```python
from build123d import *

# Parameters (mm, degrees)
PAD021_DEPTH = 7.4
PAD022_DEPTH = 10.8
SKETCH051_R  = 6.1
PAD023_DEPTH = 3.5
SKETCH052_R  = 5
PAD024_DEPTH = 4


with BuildPart() as part:
    # Sketch049 → Pad021 (new body)
    with BuildSketch(Plane.XY):
        with BuildLine():
            ThreePointArc((2.2326625821, -7.7862197371), (8.1, 0), (2.2326625821, 7.7862197371))
            Line((1.7916428128, 6.2482010236), (2.2326625821, 7.7862197371))
            ThreePointArc((1.7916428128, -6.2482010236), (6.5, 0), (1.7916428128, 6.2482010236))
            Line((1.7916428128, -6.2482010236), (2.2326625821, -7.7862197371))
        make_face()
    extrude(amount=PAD021_DEPTH)

    # Sketch050 (on Face6 of Pad021) → Pad022 (join)
    with BuildSketch(Plane.XY.offset(7.4)):
        with BuildLine():
            ThreePointArc((10.5423930727, 6.7162451043), (-12.5, 0), (10.5423930727, -6.7162451043))
            Line((10.5423930727, -6.7162451043), (7.253166434, -4.6207766318))
            ThreePointArc((7.253166434, -4.6207766318), (8.6, 0), (7.253166434, 4.6207766318))
            Line((10.5423930727, 6.7162451043), (7.253166434, 4.6207766318))
        make_face()
        with BuildLine():
            ThreePointArc((2.4256087312, 8.4591029243), (-8.8, 0), (2.4256087312, -8.4591029243))
            Line((1.7916428128, -6.2482010236), (2.4256087312, -8.4591029243))
            ThreePointArc((1.7916428128, -6.2482010236), (6.5, 0), (1.7916428128, 6.2482010236))
            Line((1.7916428128, 6.2482010236), (2.4256087312, 8.4591029243))
        make_face(mode=Mode.SUBTRACT)
    extrude(amount=PAD022_DEPTH)

    # Sketch051 (on Face10 of Pad022) → Pad023 (join)
    with BuildSketch(Plane.XY.offset(18.2)):
        with BuildLine():
            ThreePointArc((10.5423930727, 6.7162451043), (-12.5, 0), (10.5423930727, -6.7162451043))
            Line((10.5423930727, -6.7162451043), (7.253166434, -4.6207766318))
            ThreePointArc((7.253166434, -4.6207766318), (8.6, 0), (7.253166434, 4.6207766318))
            Line((10.5423930727, 6.7162451043), (7.253166434, 4.6207766318))
        make_face()
        Circle(SKETCH051_R, mode=Mode.SUBTRACT)
    extrude(amount=PAD023_DEPTH)

    # Sketch052 (on Face21 of Pad023) → Pad024 (join)
    with BuildSketch(Plane.XY.offset(21.7)):
        with BuildLine():
            ThreePointArc((10.5423930727, 6.7162451043), (-12.5, 0), (10.5423930727, -6.7162451043))
            Line((10.5423930727, -6.7162451043), (7.253166434, -4.6207766318))
            ThreePointArc((7.253166434, -4.6207766318), (8.6, 0), (7.253166434, 4.6207766318))
            Line((10.5423930727, 6.7162451043), (7.253166434, 4.6207766318))
        make_face()
        Circle(SKETCH052_R, mode=Mode.SUBTRACT)
    extrude(amount=PAD024_DEPTH)


with BuildPart() as part_1:
    # Body006 placement: moved
    add(part.part.moved(Location((0, 0, 2.2))))


solid = part_1.part
```
Check sheet for the modelled part. Datum: model origin and axes. Units: mm. A direction names the side the tool comes from. Coordinates: 2 decimals unless noted, no trailing zeros. Loops run counter-clockwise (first coordinate to the right, second up) from the corner with the lowest first, then second, coordinate; pieces in that order, holes last.
1) Sectioned sample at B-B (x = 0). Record the boundary of the cut face in (y, z).
2) Access from +Z, -Z, +X, -X, +Y, -Y to the whole of each face (thin tool, end or side, straight path). Record for faces 1 (the face through (8.1, -0.1, 5.8)), 2 (the face through (8.921, -5.683, 18.622)), 3 (the face through (6.5, -0.1, 11.2)).
3) Release check for a two-part mould opening along Y. For faces 4 (the face through (7, 0, 2.2)), 5 (the face through (8.6, -0.1, 18.6)), 6 (the face through (-12.49, 0.45, 18.62)), 7 (the face through (-6.3, -1.3, 20.4)) record: released by +Y, released by -Y, zero draft, split by the parting line, or undercut.
4) Sectioned sample at C-C (z = 12.25). Record the boundary of the cut face in (x, y).
5) Gauge pin test, flat ends, axial feed: pin 1 (8 mm diameter, centred on x = -0.5, y = 2.5, fed in from -Z); pin 2 (1.5 mm diameter, centred on x = -4, z = 20.5, fed in from -Y); pin 3 (1.5 mm diameter, centred on y = -1.5, z = 6, fed in from +X); pin 4 (6 mm diameter, centred on x = 0, y = -0.5, fed in from -Z). Record the tip position at first contact, or that the pin passes through.
6) Sectioned sample at A-A (y = 0). Record the boundary of the cut face in (x, z).
7) Sectioned sample at D-D (z = 21.25). Record the boundary of the cut face in (x, y), and give its area (3 significant figures).
8) Material ranges on probe 1 along Y at (x, z) = (0, 15); probe 2 along Y at (x, z) = (0, 26); probe 3 along X at (y, z) = (2.25, 16), recorded low to high.
Check sheet entries:
1. outline: (-12.5, 9.6) - (-8.8, 9.6) - (-8.8, 20.4) - (-6.1, 20.4) - (-6.1, 23.9) - (-5, 23.9) - (-5, 27.9) - (-12.5, 27.9) - close; (5, 23.9) - (6.1, 23.9) - (6.1, 20.4) - (8.8, 20.4) - (8.8, 9.6) - (12.5, 9.6) - (12.5, 27.9) - (5, 27.9) - close
2. face 1: -Z, +X
2. face 2: +Z, -Z, +X
2. face 3: -Z
3. face 4: zero draft
3. face 5: undercut
3. face 6: split by the parting line
3. face 7: undercut
4. outline: (7.25, -4.62) arc R8.6 ccw to (7.25, 4.62) - (10.54, 6.72) arc R12.5 ccw (long way) to (10.54, -6.72) - close; hole (1.79, -6.25) arc R6.5 ccw to (1.79, 6.25) - (2.43, 8.46) arc R8.8 ccw (long way) to (2.43, -8.46) - close
5. pin 1: stops at z = 20.4
5. pin 2: stops at y = -12.07
5. pin 3: stops at x = 8.07
5. pin 4: passes through
6. outline: (-12.5, 9.6) - (-8.8, 9.6) - (-8.8, 20.4) - (-6.1, 20.4) - (-6.1, 23.9) - (-5, 23.9) - (-5, 27.9) - (-12.5, 27.9) - close; (5, 23.9) - (6.1, 23.9) - (6.1, 20.4) - (6.5, 20.4) - (6.5, 2.2) - (8.1, 2.2) - (8.1, 9.6) - (8.6, 9.6) - (8.6, 27.9) - (5, 27.9) - close
7. outline: (7.25, -4.62) arc R8.6 ccw to (7.25, 4.62) - (10.54, 6.72) arc R12.5 ccw (long way) to (10.54, -6.72) - close; hole circle Ø12.2 at (0, 0)
7. area: 327 mm2
8. probe 1: y = -12.5 to -8.8, 8.8 to 12.5
8. probe 2: y = -12.5 to -5, 5 to 12.5
8. probe 3: x = -12.3 to -8.51, 6.1 to 8.3
